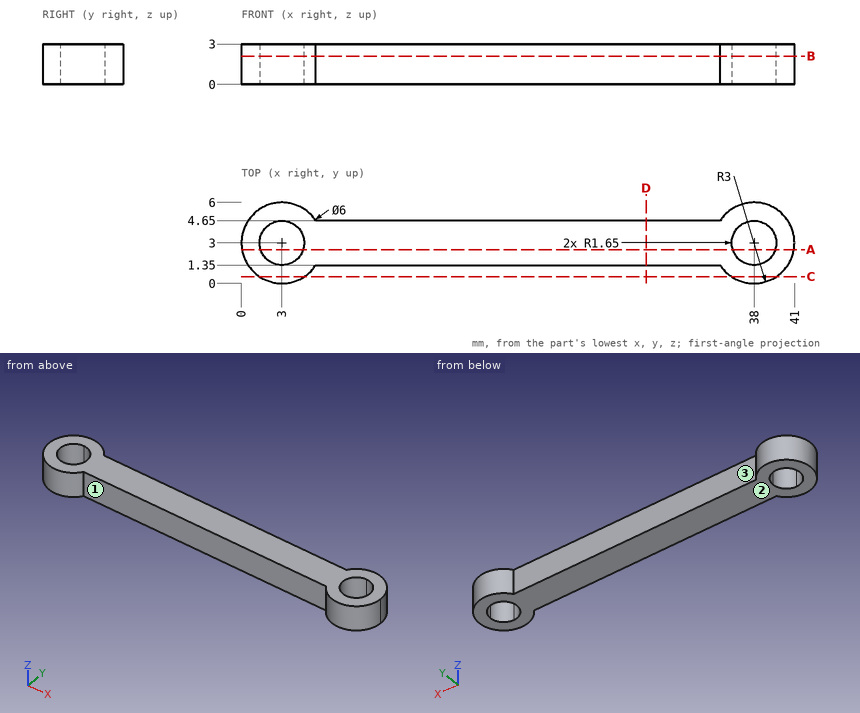
Study the drawing (mm; zero at the part's minimum x, y, z) and answer. Round coordinates to 2 decimals unless told otherwise and drop trailing zeros. Loops run counter-clockwise (first coordinate to the right, second up) from the corner with the lowest first, then second, coordinate; pieces in that order, holes last. Notation, with made-up numbers: (83.25, 1) - (137.25, 1) arc R17 cw to (137.25, 10) - close; hole circle Ø8 at (-9.75, 49.25). An arc over 180 degrees is marked (long way). Use one line per item in the form item = value. Start each with the question number.
1. The part is cut by section A-A on y = 2.5. Determine the outline of the cut face in (x, z).
2. Consider line 1 (X direction, y = 2.75, z = 0.4); line 2 (X direction, y = 4, z = 1.85); line 3 (Y direction, x = 8, z = 0.85). Determine where each line is inside the solid, lowest interval first. Write a range as [from, to].
3. The part is cut by section D-D on x = 30. Determine the outline of the cut face in (y, z), then the cut area to 3 significant figures.
4. For a pull along X with two mould halves and no side action, classify the marked faces 1, 2 and 3 as pulls with the +X half, pulls with the -X half, needs draft (parallel to the pull), parting line crosses it, or undercut.
5. Given pin 1 Ø1.5 at (x, z) = (9, 2) entering from +Y; pin 2 Ø1 at (y, z) = (2, 0.5) entering from +X, each flat-ended and moving along its own axis, determine where each tip first touches the part or whether it passes through.
6. The part is cut by section B-B on z = 2.1. Determine the outline of the cut face in (x, y), then the cut area to 3 significant figures.
7. The part is cut by section C-C on y = 0.5. Determine the outline of the cut face in (x, z).
Geometry check:
q1.outline = (0.04, 0) - (1.43, 0) - (1.43, 3) - (0.04, 3) - close; (4.57, 0) - (36.43, 0) - (36.43, 3) - (4.57, 3) - close; (39.57, 0) - (40.96, 0) - (40.96, 3) - (39.57, 3) - close
q2.line_1 = [0.01, 1.37], [4.63, 36.37], [39.63, 40.99]
q2.line_2 = [0.17, 1.69], [4.31, 36.69], [39.31, 40.83]
q2.line_3 = [1.35, 4.65]
q3.outline = (1.35, 0) - (4.65, 0) - (4.65, 3) - (1.35, 3) - close
q3.area = 9.90 mm^2
q4.face_1 = undercut
q4.face_2 = needs draft
q4.face_3 = undercut
q5.pin_1 = 4.65
q5.pin_2 = 40.96
q6.outline = (5.51, 1.35) - (35.49, 1.35) arc R3 ccw (long way) to (35.49, 4.65) - (5.51, 4.65) arc R3 ccw (long way) to start; hole circle Ø3.3 at (3, 3); hole circle Ø3.3 at (38, 3)
q6.area = 136 mm^2
q7.outline = (1.34, 0) - (4.66, 0) - (4.66, 3) - (1.34, 3) - close; (36.34, 0) - (39.66, 0) - (39.66, 3) - (36.34, 3) - close
